Work out the finished part from the listing and answer in its coordinate system (mm). A direction names the side the tool comes from. Round coordinates to 2 decimals unless told otherwise and drop trailing zeros. Loops run counter-clockwise (first coordinate to the right, second up) from the corner with the lowest first, then second, coordinate; pieces in that order, holes last. Notation, with made-up numbers: (39.5, -38) -> (97.5, -38) arc R18 ccw to (97.5, -3) -> close; hole circle Ø4 at (64.5, 34.25). An arc over 180 degrees is marked (long way). Use one line per item in the form item = value.
```python
from build123d import *

# Parameters (mm, degrees)
BOSS_EXTRUDE1_DEPTH = 63.5
SKETCH2_R           = 1.524
CUT_EXTRUDE1_DEPTH  = 67.526668337
SKETCH3_R           = 1.651
CUT_EXTRUDE2_DEPTH  = 69.314377924


with BuildPart() as part:
    # Sketch1 → Boss-Extrude1 (new body)
    with BuildSketch(Plane(origin=(0, 0, 0), x_dir=(0, 0, -1), z_dir=(1, 0, 0))):
        with BuildLine():
            Line((7.269655172, -7.62), (14.889655172, -7.62))
            Line((14.889655172, -7.62), (14.889655172, -12.7))
            Line((14.889655172, -12.7), (-0.350344828, -12.7))
            Line((-0.350344828, -12.7), (-0.350344828, 12.7))
            Line((-0.350344828, 12.7), (4.729655172, 12.7))
            Line((4.729655172, 12.7), (4.729655172, -5.08))
            ThreePointArc((4.729655172, -5.08), (5.473603948, -6.876051224), (7.269655172, -7.62))
        make_face()
    extrude(amount=BOSS_EXTRUDE1_DEPTH)

    # Sketch2 → Cut-Extrude1 (cut, through all)
    with BuildSketch(Plane.XY.offset(0.350344828)):
        with Locations((21.336, 10.16)):
            Circle(SKETCH2_R)
        with Locations((42.164, 10.16)):
            Circle(SKETCH2_R)
        with BuildLine():
            Line((10.16, 0), (10.16, -12.7))
            Line((10.16, -12.7), (53.34, -12.7))
            Line((53.34, -12.7), (53.34, 0))
            ThreePointArc((53.34, 0), (51.108153673, 5.388153673), (45.72, 7.62))
            Line((45.72, 7.62), (17.78, 7.62))
            ThreePointArc((17.78, 7.62), (12.391846327, 5.388153673), (10.16, 0))
        make_face()
    extrude(amount=-CUT_EXTRUDE1_DEPTH, mode=Mode.SUBTRACT)

    # Sketch3 → Cut-Extrude2 (cut, through all)
    with BuildSketch(Plane(origin=(0, -7.62, 0), x_dir=(1, 0, 0), z_dir=(0, 1, 0))):
        with Locations(Location((5.08, 11.587655172, 0), (0, 0, 270))):
            Circle(SKETCH3_R)
        with Locations(Location((58.42, 11.587655172, 0), (0, 0, 270))):
            Circle(SKETCH3_R)
    extrude(amount=-CUT_EXTRUDE2_DEPTH, mode=Mode.SUBTRACT)


solid = part.part
```
(1) Given P1, Ø3, axis at x = 52.5, z = -5.5, coming from the -Y side; P2, Ø3.5, axis at x = 42.164, y = 10.16, coming from the -Z side; P3, Ø5, axis at x = 33, z = -3.5, coming from the -Y side; P4, Ø4, axis at x = 2.5, z = -12.5, coming from the +Y side, each flat-ended and moving along its own axis, determine where each tip first touches the part or whether it passes through.
Completed:
P1 = -12.7
P2 = -4.73
P3 = 7.62
P4 = -7.62
(2) Find section A-A, the plane z = -8.5. Write down the section's boundary in (x, y), then the cut area to 3 significant figures.
Completed:
outline = (0, -12.7) -> (10.16, -12.7) -> (10.16, -7.62) -> (0, -7.62) -> close; (53.34, -12.7) -> (63.5, -12.7) -> (63.5, -7.62) -> (53.34, -7.62) -> close
area = 103 mm2
(3) Find section B-B, the plane y = -1.75. Write down the section's boundary in (x, z), then the cut area to 3 significant figures.
Completed:
outline = (0, -4.73) -> (10.16, -4.73) -> (10.16, 0.35) -> (0, 0.35) -> close; (53.34, -4.73) -> (63.5, -4.73) -> (63.5, 0.35) -> (53.34, 0.35) -> close
area = 103 mm2
(4) Consider L1, parallel to Y at x = 35, z = -2.25; L2, parallel to Z at x = 58.5, y = 9.25; L3, parallel to X at y = -3, z = -1. Determine where each line is inside the solid, lowest interval first.
Completed:
L1 = 7.62 to 12.7
L2 = -4.73 to 0.35
L3 = 0 to 10.16, 53.34 to 63.5
(5) For faces 1 (the cylindrical face through (60.057, -10.124, -11.803)), 2 (the flat face through (4, -7.62, -10)), 3 (the flat face through (32, 7.62, -2)), determine the directions among +Z, -Z, +X, -X, +Y, -Y from which every point of the face is accessible in a straight line to the end or side of a thin tool.
Completed:
face_1 = +Y, -Y
face_2 = -Z, +X, -X, +Y
face_3 = +Z, -Z, -Y
(6) Find section D-D, the plane z = -1. Write down the section's boundary in (x, y).
Completed:
outline = (0, -12.7) -> (10.16, -12.7) -> (10.16, 0) arc R7.62 cw to (17.78, 7.62) -> (45.72, 7.62) arc R7.62 cw to (53.34, 0) -> (53.34, -12.7) -> (63.5, -12.7) -> (63.5, 12.7) -> (0, 12.7) -> close; hole circle Ø3.05 at (21.34, 10.16); hole circle Ø3.05 at (42.16, 10.16)
(7) Find section C-C, the plane y = 10.16. Write down the section's boundary in (x, z), then the cut area to 3 significant figures.
Completed:
outline = (0, -4.73) -> (19.81, -4.73) -> (19.81, 0.35) -> (0, 0.35) -> close; (22.86, -4.73) -> (40.64, -4.73) -> (40.64, 0.35) -> (22.86, 0.35) -> close; (43.69, -4.73) -> (63.5, -4.73) -> (63.5, 0.35) -> (43.69, 0.35) -> close
area = 292 mm2
(8) For a pull along Z with two mould halves and no side action, classify faces 4 (the flat face through (10.16, -8, -5)), 5 (the cylindrical face through (5, -6.9, -5.5)), 6 (the cylindrical face through (3.47, -10.12, -11.95)) as +Z half, -Z half, draft (parallel to the pull), parting line (faces both ways), or undercut.
Completed:
face_4 = draft
face_5 = -Z half
face_6 = undercut
